Autodesk Inventor part; units mm, degrees
ref_plane "YZ Plane" through (0, 0, 0) normal (1, 0, 0) x (0, 1, 0)
ref_plane "XZ Plane" through (0, 0, 0) normal (0, 1, 0) x (-1, 0, 0)
ref_plane "XY Plane" through (0, 0, 0) normal (0, 0, 1) x (1, 0, 0)
sketch "スケッチ1" plane through (0, 0, 0) normal (1, 0, 0) x (0, 1, 0)
  line L0 (3.7, 0) -> (-3.7, 0)
  line L1 (-3.7, 0) -> (-3.7, -3)
  line L2 (-3.7, -3) -> (3.7, -3)
  line L3 (3.7, -3) -> (3.7, 0)
  line L4 (2.5, -3) -> (-2.5, -3)
  line L5 (-2.5, -3) -> (-2.5, -11.5)
  line L6 (-2.5, -11.5) -> (2.5, -11.5)
  line L7 (2.5, -11.5) -> (2.5, -3)
  point P0 (0, 0)
  point P1 (0, 0)
  point P2 (0, -3)
  dimension "d0" = 7.4
  dimension "d1" = 3
  dimension "d2" = 5
  dimension "d3" = 8.5
extrude "押し出し1" add sketch "スケッチ1" along normal blind 0.5
sketch "スケッチ2" plane through (0.5, 0, 0) normal (1, 0, 0) x (0, 0, -1)
  ellipse E0 centre (8, 0) end of major axis (9.5, 0) minor radius 1.3
  line L0 (0, 3.7) -> (0, -3.7)
  line L1 (11.5, -2.5) -> (11.5, 2.5)
  point P0 (0, 0)
  point P1 (0, 0)
  dimension "d6" = 1.3
  dimension "d7" = 1.5
  dimension "d8" = 3.5
extrude "押し出し2" cut sketch "スケッチ2" against normal through all
fillet "フィレット1" radius 0.5 2 edges at (0.25, -2.5, -11.5) (0.25, 2.5, -11.5)
properties part number "555_Terminal" material "銅"
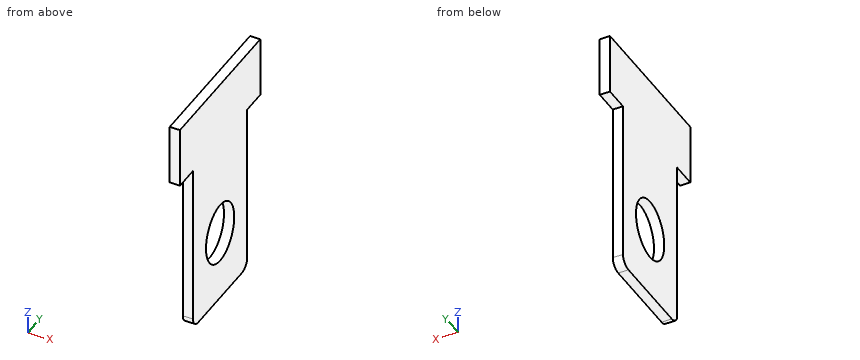
CAD build for the part. Positions are in the model's coordinates, mm. Give positions to 0.01 mm unless a question says otherwise; leave off trailing zeros. Loops run counter-clockwise (first coordinate to the right, second up) from the corner with the lowest first, then second, coordinate; pieces in that order, holes last. Notation, with made-up numbers: (86.25, 70) -> (96.25, 70) arc R24 ccw to (96.25, 96) -> close; hole circle Ø10 at (-36, -36). An arc over 180 degrees is marked (long way). Use a Markdown table: item, result.
1. Slice it at A-A (z = -4). List the corners of the cut face in (x, y), plus the area to 3 significant figures.
Check result:
| item | result |
|---|---|
| outline | (0, -2.5) -> (0.5, -2.5) -> (0.5, 2.5) -> (0, 2.5) -> close |
| area | 2.50 mm^2 |
2. Slice it at B-B (y = -3). List the corners of the cut face in (x, z).
Check result:
| item | result |
|---|---|
| outline | (0, -3) -> (0.5, -3) -> (0.5, 0) -> (0, 0) -> close |
3. Flat gauge pin, fed straight in: pin 1 (1 mm diameter, centred on y = -2, z = -5, fed in from -X). Where does the tip first touch, or does it go through?
Check result:
| item | result |
|---|---|
| pin 1 | stops at x = 0 |
4. Wall check: L1, parallel to Y at x = 0.4, z = -5.5; L2, parallel to Z at x = 0.35, y = -3.5; L3, parallel to Y at x = 0.25, z = -9.25. Give the ranges that are in metal, low to high. Write a range as [from, to].
Check result:
| item | result |
|---|---|
| L1 | y = [-2.5, 2.5] |
| L2 | z = [-3, 0] |
| L3 | y = [-2.5, -0.72], [0.72, 2.5] |
